```python
from build123d import *

# Parameters (mm, degrees)
SKETCH1_R           = 44.5
BOSS_EXTRUDE1_DEPTH = 10
SKETCH2_R           = 37
BOSS_EXTRUDE2_DEPTH = 10
CUT_EXTRUDE1_DEPTH  = 67.034082109


with BuildPart() as part:
    # Sketch1 → Boss-Extrude1 (new body)
    with BuildSketch(Plane(origin=(0, 0, 0), x_dir=(1, 0, 0), z_dir=(0, 1, 0))):
        with Locations(Location((0, 0, 0), (0, 0, 270))):
            Circle(SKETCH1_R)
    extrude(amount=BOSS_EXTRUDE1_DEPTH)

    # Sketch2 → Boss-Extrude2 (add)
    with BuildSketch(Plane(origin=(0, 10, 0), x_dir=(1, 0, 0), z_dir=(0, 1, 0))):
        with Locations(Location((0, 0, 0), (0, 0, 270))):
            Circle(SKETCH2_R)
    extrude(amount=BOSS_EXTRUDE2_DEPTH)

    # Sketch3 → Cut-Extrude1 (cut, through all)
    with BuildSketch(Plane.XZ):
        with BuildLine():
            Line((-13, 0), (-13, 42.558782877))
            Line((-13, 42.558782877), (-13, 62.217124748))
            Line((-13, 62.217124748), (13, 62.217124748))
            Line((13, 62.217124748), (13, 0))
            ThreePointArc((13, 0), (0, -13), (-13, 0))
        make_face()
    extrude(amount=-CUT_EXTRUDE1_DEPTH, mode=Mode.SUBTRACT)


solid = part.part
```
Can you work these out from the model? Positions are in its coordinate system, mm. A direction names the side the tool comes from. Round coordinates to 2 decimals unless told otherwise and drop trailing zeros. Loops run counter-clockwise (first coordinate to the right, second up) from the corner with the lowest first, then second, coordinate; pieces in that order, holes last. Notation, with made-up numbers: M -9,60 L 23,60 A4 cw 23,66 Z; hole C 46.5,66.5 d9. An arc over 180 degrees is marked long. Answer in a Markdown table with one row per item.
1. Thinking about a two-plate mould opening in X: for faces 4 (the face through (13, 10, 22)), 5 (the face through (7, 10, -37)), 6 (the face through (1.772, 4.93, -44.465)), which applies, pulls with the +X half, pulls with the -X half, needs draft (parallel to the pull), parting line crosses it, or undercut?
Established:
| item | result |
|---|---|
| face 4 | undercut |
| face 5 | needs draft |
| face 6 | parting line crosses it |
2. If we section it at B-B, the plane z = -3.5: Please give me the cut outline in (x, y).
Established:
| item | result |
|---|---|
| outline | M -44.36,0 L -12.52,0 L -12.52,20 L -36.83,20 L -36.83,10 L -44.36,10 Z; M 12.52,0 L 44.36,0 L 44.36,10 L 36.83,10 L 36.83,20 L 12.52,20 Z |
3. If we section it at A-A, the plane x = 0: Please give me the cut outline in (y, z).
Established:
| item | result |
|---|---|
| outline | M 0,-44.5 L 10,-44.5 L 10,-37 L 20,-37 L 20,-13 L 0,-13 Z |
4. On a 3-axis mill with a long thin cutter (end or side, diameter ignored), from which of +Z, -Z, +X, -X, +Y, -Y can I reach the whole of each face in a straight line? I mean faces 1 (the face through (1.44, 14.93, -36.97)), 2 (the face through (-13, 10, 21)), 3 (the face through (9, 20, -10)). Say none if no direction works.
Established:
| item | result |
|---|---|
| face 1 | +Y |
| face 2 | +Z, +Y, -Y |
| face 3 | +Z, -Z, +X, -X, +Y |
5. If we section it at C-C, the plane z = 11: Please give me the cut outline in (x, y).
Established:
| item | result |
|---|---|
| outline | M -43.12,0 L -13,0 L -13,20 L -35.33,20 L -35.33,10 L -43.12,10 Z; M 13,0 L 43.12,0 L 43.12,10 L 35.33,10 L 35.33,20 L 13,20 Z |
6. I'm going to push flat-ended pins straight in: pin 1 Ø4 at (x, y) = (26.5, 13.5) entering from -Z; pin 2 Ø6 at (y, z) = (15, 24.5) entering from -X; pin 3 Ø8 at (x, y) = (-29.5, 11) entering from -Z. Where does each tip first touch, or does it pass through?
Established:
| item | result |
|---|---|
| pin 1 | z = -27.73 |
| pin 2 | x = -30.11 |
| pin 3 | z = -36.38 |
7. If we section it at D-D, the plane x = -33: Please give me the cut outline in (y, z), plus the area to 3 significant figures.
Established:
| item | result |
|---|---|
| outline | M 0,-29.85 L 10,-29.85 L 10,-16.73 L 20,-16.73 L 20,16.73 L 10,16.73 L 10,29.85 L 0,29.85 Z |
| area | 932 mm² |
8. Please list where these lines run through material, in increasing order: line 1 (X direction, y = 19.25, z = 23); line 2 (X direction, y = 13.25, z = 30); line 3 (Y direction, x = 14, z = -36.5). Write a range as from..to.
Established:
| item | result |
|---|---|
| line 1 | -28.98..-13, 13..28.98 |
| line 2 | -21.66..-13, 13..21.66 |
| line 3 | 0..10 |
